Verification items for the finished model (mm, model axes). A direction names the side the tool comes from. Coordinates: 2 decimals unless noted, no trailing zeros. Write each loop counter-clockwise with the first axis right and the second up, starting at its lowest first coordinate (ties: lowest second). Pieces come first, ordered by that corner, then holes. Notation, with made-up numbers: M 50,71.25 L 66,71.25 A13 ccw 66,81.25 Z; hole C 30,-5 d11. An arc over 180 degrees is marked long. One line per item, written item: value.
```python
from build123d import *

# Parameters (mm, degrees)
SKETCH1_R           = 5.0038
BOSS_EXTRUDE1_DEPTH = 1.6002
SKETCH2_R           = 2.38125
BOSS_EXTRUDE2_DEPTH = 14.605
FILLET1_R           = 2.54


with BuildPart() as part:
    # Sketch1 → Boss-Extrude1 (new body)
    with BuildSketch(Plane.XY):
        Circle(SKETCH1_R)
    extrude(amount=BOSS_EXTRUDE1_DEPTH)

    # Sketch2 → Boss-Extrude2 (add)
    with BuildSketch(Plane.XY):
        Circle(SKETCH2_R)
    extrude(amount=-BOSS_EXTRUDE2_DEPTH)

    # Fillet1
    # the kernel refuses this fillet: 2.54 mm, written as the material it takes off along each edge
    with BuildSketch(Plane(origin=(0, 0, 1.6002), x_dir=(1, 0, 0), z_dir=(0, -1, 0))) as fillet1_piece_1:
        with BuildLine():
            CenterArc((2.644059345, -2.54), FILLET1_R, 21.715617283, 68.284382717)
            Line((2.644059345, 0), (2.644059345, 0.0508))
            Line((2.644059345, 0.0508), (5.0038, 0.0508))
            Line((5.0038, 0.0508), (5.0546, 0))
            ThreePointArc((5.0546, 0), (5.0546, -0.8001), (5.050994813, -1.581404))
            Line((5.050994813, -1.581404), (5.0038, -1.6002))
        make_face()
    revolve(axis=Axis((0, 0, 1.6002), (0, 0, 1)), mode=Mode.SUBTRACT)


solid = part.part
```
Item 1: Cross-section at C-C, the plane z = -1.75. Enter the section's corners in (x, y).
The answers:
outline: C 0,0 d4.76
Item 2: Cross-section at A-A, the plane x = 0. Enter the section's corners in (y, z) (3 decimals).
The answers:
outline: M -5.004,0 L -2.381,0 L -2.381,-14.605 L 2.381,-14.605 L 2.381,0 L 5.004,0 A2.54 ccw 2.644,1.6 L -2.644,1.6 A2.54 ccw Z
Item 3: Go/stop test with flat-tipped pins: P1, Ø2, axis at y = -1, z = -5, coming from the -X side; P2, Ø1.5, axis at y = 4, z = -7.5, coming from the +X side; P3, Ø3, axis at x = 2, z = -3, coming from the +Y side. Record where each tip stops, or that it passes through.
The answers:
P1: stops at x = -2.38
P2: passes through
P3: stops at y = 2.33
Item 4: Scan lines: line 1 (Y direction, x = 0, z = -4.75); line 2 (Z direction, x = -0.75, y = 2.5); line 3 (Z direction, x = 4.25, y = -0.75). Record each from-to range of solid material in increasing order.
The answers:
line 1: y = -2.38 to 2.38
line 2: z = 0 to 1.6
line 3: z = 0 to 0.97
Item 5: Access from +Z, -Z, +X, -X, +Y, -Y to the whole of each face (thin tool, end or side, straight path). Record for faces 1 (the face through (-1.89, -1.45, -7.2)), 2 (the face through (0, 0, 1.6)).
The answers:
face 1: -Z
face 2: +Z, +X, -X, +Y, -Y
